For this review, take the finished solid that the model builds, in its own axes (mm). A direction names the side the tool comes from. Coordinates: 2 decimals unless noted, no trailing zeros. Order: outer loops, then holes, each group sorted by start corner. A loop starts at its lowest first (then second) coordinate and runs counter-clockwise, first axis right, second up. Notation, with made-up numbers: (-3, -3.5) -> (40, -3.5) arc R32 cw to (40, 22.5) -> close; hole circle Ø1 at (69.5, -27.5). An arc over 180 degrees is marked (long way). Return JSON: item names as keys, results as strings. Group by question number.
Item 1: Machinability: for faces 1 (the flat face through (0, -13, -19.05)), 2 (the flat face through (-19.05, -13, 0)), 3 (the flat face through (0, -13, 19.05)), which of the approach directions +Z, -Z, +X, -X, +Y, -Y give a long, thin tool a straight path to every point of the face, cutting with its end or side? Answer none if there is none.
Item 2: Take a section at B-B (z = 0). Write out the cut boundary in (x, y).
Item 3: Insertion check: pin 1 (6 mm diameter, centred on x = 13, y = -5.5, fed in from -Z); pin 2 (20.5 mm diameter, centred on y = -13.5, z = 1.5, fed in from +X). Each pin has a flat end and moves straight along its axis. Give the tip position at first contact, or say it passes through.
Item 4: Take a section at C-C (x = 17). Write out the cut boundary in (y, z), then the cut area to 3 significant figures.
Item 5: Take a section at A-A (x = 0). Write out the cut boundary in (y, z), then the cut area to 3 significant figures.
Item 6: Draft analysis for pull direction X (two halves, no side actions). For faces 4 (the flat face through (-1, 0, -20)), 5 (the flat face through (19.05, -13, 0)), 6 (the cylindrical face through (-6.827, 48.809, -4.487)), state which applies: +X half, -X half, draft (parallel to the pull), parting line (faces both ways), or undercut.
Item 7: For line 1 along X through (y, z) = (38, -22); line 2 along Y through (x, z) = (0, 17); line 3 along X through (y, z) = (69.5, 9.5), list the stretches that pass through material, from the lowest coordinate up.
Item 8: Take a section at D-D (y = 38.1). Write out the cut boundary in (x, z), then the cut area to 3 significant figures.
```python
from build123d import *

# Parameters (mm, degrees)
F0_W     = 76.2
F0_H     = 76.2
F1_DEPTH = 76.2
F3_D     = 25.4
F4_W     = 38.1
F4_H     = 38.1
F5_DEPTH = 25.4
F6_R     = 12.7
F7_DEPTH = 12.7


with BuildPart() as f1:
    # F0 (on Front) → F1 (new body)
    with BuildSketch(Plane.XZ):
        with Locations((0, -3.953981)):
            Rectangle(F0_W, F0_H)
    extrude(amount=-F1_DEPTH)

    # F3 (through all)
    with Locations(Plane.XY.offset(34.146019)):
        with Locations((0, 38.1)):
            Hole(F3_D / 2)

    # F4 (on face) → F5 (join)
    with BuildSketch(Plane.XZ):
        Rectangle(F4_W, F4_H)
    extrude(amount=F5_DEPTH)

    # F6 (on face) → F7 (join)
    with BuildSketch(Plane.YZ.offset(38.1)):
        with Locations((39.500758, 0)):
            Circle(F6_R)
    extrude(amount=F7_DEPTH)


solid = f1.part
```
Findings below:
{
 "1": {"face 1": "-Z, +X, -X, -Y", "face 2": "+Z, -Z, -X, -Y", "face 3": "+Z, +X, -X, -Y"},
 "2": {"outline": "(-38.1, 0) -> (-19.05, 0) -> (-19.05, -25.4) -> (19.05, -25.4) -> (19.05, 0) -> (38.1, 0) -> (38.1, 26.8) -> (50.8, 26.8) -> (50.8, 52.2) -> (38.1, 52.2) -> (38.1, 76.2) -> (-38.1, 76.2) -> close; hole circle Ø25.4 at (0, 38.1)"},
 "3": {"pin 1": "stops at z = -19.05", "pin 2": "stops at x = 19.05"},
 "4": {"outline": "(-25.4, -19.05) -> (0, -19.05) -> (0, -42.05) -> (76.2, -42.05) -> (76.2, 34.15) -> (0, 34.15) -> (0, 19.05) -> (-25.4, 19.05) -> close", "area": "6,770 mm2"},
 "5": {"outline": "(-25.4, -19.05) -> (0, -19.05) -> (0, -42.05) -> (25.4, -42.05) -> (25.4, 34.15) -> (0, 34.15) -> (0, 19.05) -> (-25.4, 19.05) -> close; (50.8, -42.05) -> (76.2, -42.05) -> (76.2, 34.15) -> (50.8, 34.15) -> close", "area": "4,840 mm2"},
 "6": {"face 4": "draft", "face 5": "+X half", "face 6": "undercut"},
 "7": {"line 1": "x = -38.1 to -12.7, 12.7 to 38.1", "line 2": "y = -25.4 to 25.4, 50.8 to 76.2", "line 3": "x = -38.1 to 38.1"},
 "8": {"outline": "(-38.1, -42.05) -> (-12.7, -42.05) -> (-12.7, 34.15) -> (-38.1, 34.15) -> close; (12.7, -42.05) -> (38.1, -42.05) -> (38.1, -12.62) -> (50.8, -12.62) -> (50.8, 12.62) -> (38.1, 12.62) -> (38.1, 34.15) -> (12.7, 34.15) -> close", "area": "4,190 mm2"}
}
